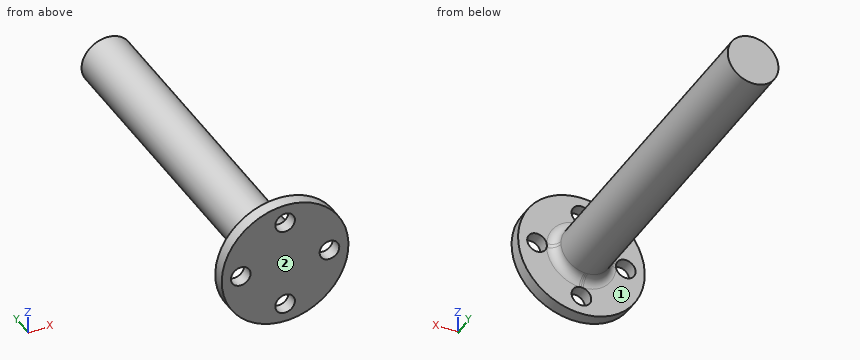
from build123d import *

# Parameters (mm, degrees)
SKETCH_1_R          = 10
EXTRUDE_1_DEPTH     = 2
SKETCH_2_R          = 1.55
CUT_EXTRUDE_1_DEPTH = 2
SKETCH_3_R          = 4
EXTRUDE_2_DEPTH     = 53
FILLET_1_R          = 1.5


with BuildPart() as part:
    # 草图1 → 凸台-拉伸1 (new body)
    with BuildSketch(Plane(origin=(0, 0, 0), x_dir=(1, 0, 0), z_dir=(0, 1, 0))):
        with Locations(Location((0, 0, 0), (0, 0, 270))):
            Circle(SKETCH_1_R)
    extrude(amount=EXTRUDE_1_DEPTH)

    # 草图2 → 切除-拉伸1 (cut)
    with BuildSketch(Plane(origin=(0, 2, 0), x_dir=(1, 0, 0), z_dir=(0, 1, 0))):
        with Locations(Location((0, 7, 0), (0, 0, 270))):
            Circle(SKETCH_2_R)
        with Locations(Location((7, 0, 0), (0, 0, 270))):
            Circle(SKETCH_2_R)
        with Locations(Location((-7, 0, 0), (0, 0, 270))):
            Circle(SKETCH_2_R)
        with Locations(Location((0, -7, 0), (0, 0, 270))):
            Circle(SKETCH_2_R)
    extrude(amount=-CUT_EXTRUDE_1_DEPTH, mode=Mode.SUBTRACT)

    # 草图3 → 凸台-拉伸2 (add)
    with BuildSketch(Plane(origin=(0, 2, 0), x_dir=(1, 0, 0), z_dir=(0, 1, 0))):
        with Locations(Location((0, 0, 0), (0, 0, 270))):
            Circle(SKETCH_3_R)
    extrude(amount=EXTRUDE_2_DEPTH)

    # 圆角1
    fillet_1_edges = [part.edges().sort_by_distance(p)[0] for p in [
        (0, 2, -4),
    ]]
    fillet(fillet_1_edges, radius=FILLET_1_R)


solid = part.part
Geometry: final body of the model. Coordinates: model frame, mm. Face numbers are marked on the shaded views. A direction names the side the tool comes from. Coordinates: 2 decimals unless noted, no trailing zeros. Loops run counter-clockwise (first coordinate to the right, second up) from the corner with the lowest first, then second, coordinate; pieces in that order, holes last. Notation, with made-up numbers: (52.25, 23) - (70.25, 23) arc R21 ccw to (70.25, 56) - close; hole circle Ø5 at (79, -25.5). An arc over 180 degrees is marked (long way). One line per question, with ' | ' between items. Start each with the question number.
(1) Cut plane B-B on y = 44. Output: boundary loops of the cut face in (x, z), and give its area (3 significant figures).
(2) Cut plane A-A on z = 7.25. Output: boundary loops of the cut face in (x, y).
(3) Reachability of the marked faces 1 and 2 from +Z, -Z, +X, -X, +Y, -Y: full face, straight path, thin tool, end or side. Return the list, or none.
(4) Ray query, L1, parallel to X at y = 1, z = 0; L2, parallel to Z at x = -7, y = 0.9. Return the intervals inside material, ascending. Write a range as from..to.
(5) First-contact query: pin 1 (3.5 mm diameter, centred on x = 7, z = 0, fed in from -Y); pin 2 (3 mm diameter, centred on y = 29, z = -1, fed in from +X); pin 3 (8 mm diameter, centred on y = 30.5, z = -2.5, fed in from -X); pin 4 (1 mm diameter, centred on y = 44, z = -3.5, fed in from -X). Flat tips, straight axial feed; report the tip coordinate or a pass-through.
(6) Cut plane C-C on z = -7.5. Output: boundary loops of the cut face in (x, y).
Here are the results:
1) outline: circle Ø8 at (0, 0) | area: 50.3 mm²
2) outline: (-6.89, 0) - (-1.53, 0) - (-1.53, 2) - (-6.89, 2) - close; (1.53, 0) - (6.89, 0) - (6.89, 2) - (1.53, 2) - close
3) face 1: +Y | face 2: +Z, -Z, +X, -X, -Y
4) L1: -10..-8.55, -5.45..5.45, 8.55..10 | L2: -7.14..-1.55, 1.55..7.14
5) pin 1: y = 0 | pin 2: x = 4 | pin 3: x = -4 | pin 4: x = -2.65
6) outline: (-6.61, 0) - (-1.47, 0) - (-1.47, 2) - (-6.61, 2) - close; (1.47, 0) - (6.61, 0) - (6.61, 2) - (1.47, 2) - close
